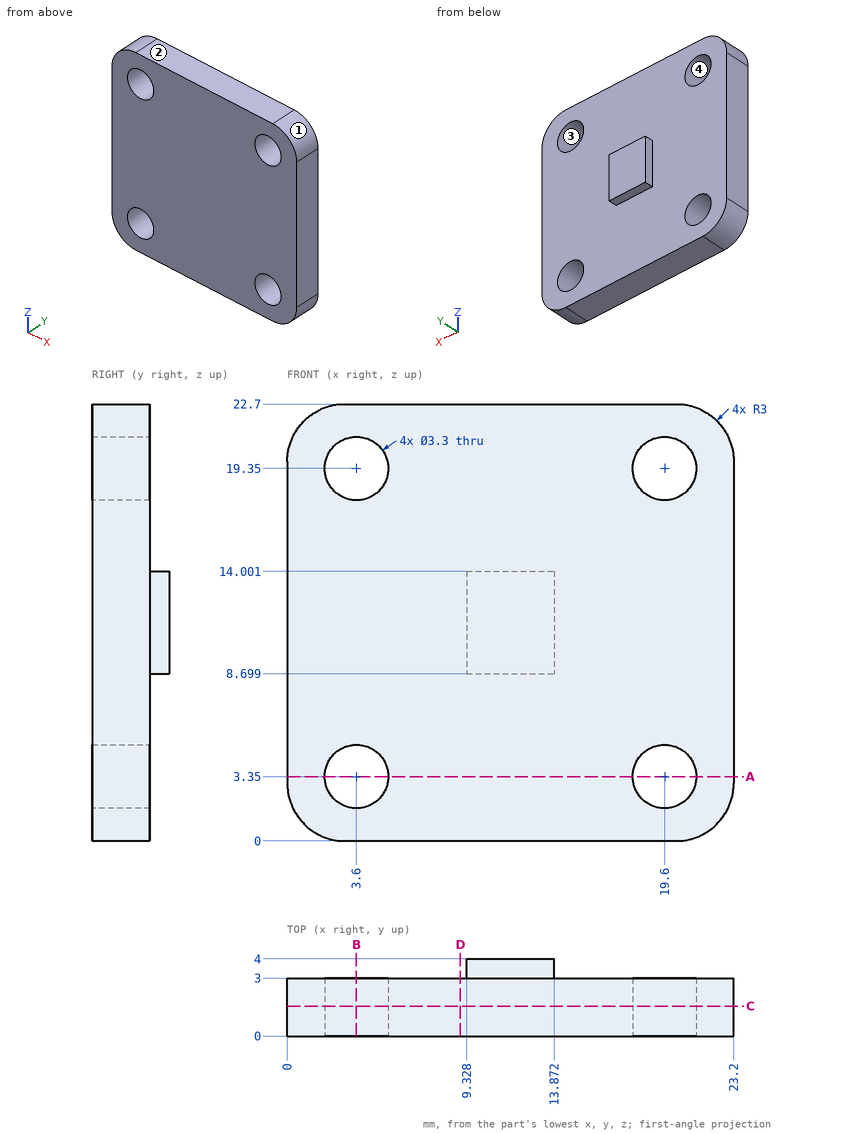
Input: dimensioned drawing with shaded views. Units: mm. Origin: part minimum x, y, z. Round coordinates to 2 decimals unless told otherwise and drop trailing zeros. Loops run counter-clockwise (first coordinate to the right, second up) from the corner with the lowest first, then second, coordinate; pieces in that order, holes last. Notation, with made-up numbers: M 24,71.25 L 50,71.25 A31 ccw 50,96.25 Z; hole C 55,-38.5 d9. An arc over 180 degrees is marked long. Answer in a Markdown table with one row per item. Add a question column.
1. Section B-B (x = 3.6). Output: boundary loops of the cut face in (y, z), and give its area (3 significant figures).
2. Ray query, probe 1 along X at (y, z) = (1.8, 3.35); probe 2 along Y at (x, z) = (2, 1); probe 3 along X at (y, z) = (0.2, 20.25). Return the intervals inside material, ascending.
3. Contact query for flat-ended pins moving along their axis: pin 1 (0.8 mm diameter, centred on x = 12.5, y = 3.5, fed in from +Z); pin 2 (0.8 mm diameter, centred on x = 11, y = 3.5, fed in from -Z); pin 3 (4 mm diameter, centred on x = 3.6, z = 19.35, fed in from +Y). Output: stop coordinate, or through.
4. Section C-C (y = 1.55). Output: boundary loops of the cut face in (x, z).
5. Section D-D (x = 9). Output: boundary loops of the cut face in (y, z), and give its area (3 significant figures).
6. Section A-A (z = 3.35). Output: boundary loops of the cut face in (x, y), and give its area (3 significant figures).
7. Mould query, pull axis X, two halves, no side actions, for the marked faces 1, 2, 3 and 4. Classes: released by +X, released by -X, zero draft, split by the parting line, or undercut.
Values follow:
| question | item | result |
|---|---|---|
| 1 | outline | M 0,0 L 3,0 L 3,1.7 L 0,1.7 Z; M 0,5 L 3,5 L 3,17.7 L 0,17.7 Z; M 0,21 L 3,21 L 3,22.7 L 0,22.7 Z |
| 1 | area | 48.3 mm^2 |
| 2 | probe 1 | 0 to 1.95, 5.25 to 17.95, 21.25 to 23.2 |
| 2 | probe 2 | 0 to 3 |
| 2 | probe 3 | 0.05 to 2.22, 4.98 to 18.22, 20.98 to 23.15 |
| 3 | pin 1 | z = 14 |
| 3 | pin 2 | z = 8.7 |
| 3 | pin 3 | y = 3 |
| 4 | outline | M 0,3 A3 ccw 3,0 L 20.2,0 A3 ccw 23.2,3 L 23.2,19.7 A3 ccw 20.2,22.7 L 3,22.7 A3 ccw 0,19.7 Z; hole C 3.6,3.35 d3.3; hole C 3.6,19.35 d3.3; hole C 19.6,3.35 d3.3; hole C 19.6,19.35 d3.3 |
| 5 | outline | M 0,0 L 3,0 L 3,22.7 L 0,22.7 Z |
| 5 | area | 68.1 mm^2 |
| 6 | outline | M 0,0 L 1.95,0 L 1.95,3 L 0,3 Z; M 5.25,0 L 17.95,0 L 17.95,3 L 5.25,3 Z; M 21.25,0 L 23.2,0 L 23.2,3 L 21.25,3 Z |
| 6 | area | 49.8 mm^2 |
| 7 | face 1 | released by +X |
| 7 | face 2 | zero draft |
| 7 | face 3 | undercut |
| 7 | face 4 | undercut |
